```python
from build123d import *

# Parameters (mm, degrees)
SKETCH1_R           = 2.95
SKETCH1_R_2         = 1.9
BOSS_EXTRUDE1_DEPTH = 2
SKETCH2_R           = 0.5000000000000008
SKETCH2_R_2         = 0.75
BOSS_EXTRUDE2_DEPTH = 1.7


with BuildPart() as part:
    # Sketch1 → Boss-Extrude1 (new body)
    with BuildSketch(Plane(origin=(0, 0, 0), x_dir=(1, 0, 0), z_dir=(0, 1, 0))):
        with Locations(Location((0, 0, 0), (0, 0, 270))):
            Circle(SKETCH1_R)
        with Locations(Location((0, 0, 0), (0, 0, 270))):
            Circle(SKETCH1_R_2, mode=Mode.SUBTRACT)
    extrude(amount=BOSS_EXTRUDE1_DEPTH)

    # Sketch2 → Boss-Extrude2 (add)
    with BuildSketch(Plane(origin=(0, 2, 0), x_dir=(1, 0, 0), z_dir=(0, 1, 0))):
        with BuildLine():
            Line((-0.3719565217391307, 2.9264566195205663), (-11.689130434782609, 1.488028789586728))
            ThreePointArc((-11.689130434782609, 1.488028789586728), (-13, 1.8e-16), (-11.689130434782609, -1.488028789586728))
            Line((-11.689130434782609, -1.488028789586728), (-0.3719565217391307, -2.9264566195205663))
            ThreePointArc((-0.3719565217391307, -2.9264566195205663), (1.8e-16, -2.9500000000000024), (0.3719565217391307, -2.9264566195205663))
            Line((0.3719565217391307, -2.9264566195205663), (11.689130434782609, -1.488028789586728))
            ThreePointArc((11.689130434782609, -1.488028789586728), (13, 0), (11.689130434782609, 1.488028789586728))
            Line((11.689130434782609, 1.488028789586728), (0.3719565217391307, 2.9264566195205663))
            ThreePointArc((0.3719565217391307, 2.9264566195205663), (1.8e-16, 2.9500000000000024), (-0.3719565217391307, 2.9264566195205663))
        make_face()
        with Locations(Location((-11.5, 0, 0), (0, 0, 270))):
            Circle(SKETCH2_R, mode=Mode.SUBTRACT)
        with Locations(Location((-9.5, 0, 0), (0, 0, 270))):
            Circle(SKETCH2_R, mode=Mode.SUBTRACT)
        with Locations(Location((-7.5, 0, 0), (0, 0, 270))):
            Circle(SKETCH2_R, mode=Mode.SUBTRACT)
        with Locations(Location((7.5, 0, 0), (0, 0, 90))):
            Circle(SKETCH2_R, mode=Mode.SUBTRACT)
        with Locations(Location((9.5, 0, 0), (0, 0, 90))):
            Circle(SKETCH2_R, mode=Mode.SUBTRACT)
        with Locations(Location((11.5, 0, 0), (0, 0, 90))):
            Circle(SKETCH2_R, mode=Mode.SUBTRACT)
        with Locations(Location((0, 0, 0), (0, 0, 270))):
            Circle(SKETCH2_R_2, mode=Mode.SUBTRACT)
    extrude(amount=BOSS_EXTRUDE2_DEPTH)


solid = part.part
```
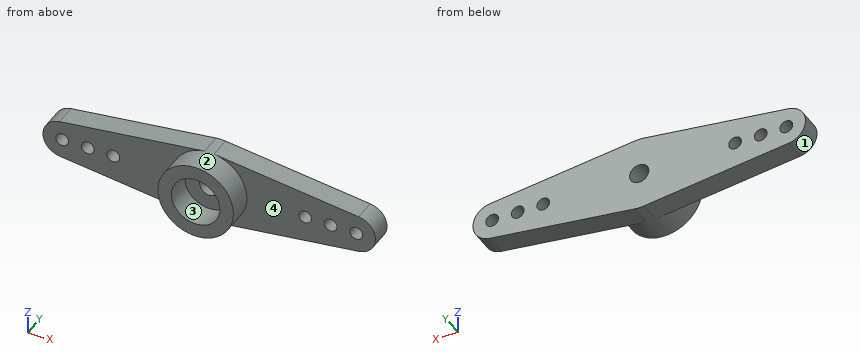
Part model, mm, in its own coordinate system. Face numbers are marked on the shaded views. Round coordinates to 2 decimals unless told otherwise and drop trailing zeros. Order: outer loops, then holes, each group sorted by start corner. A loop starts at its lowest first (then second) coordinate and runs counter-clockwise, first axis right, second up. Notation, with made-up numbers: M 39,71.25 L 66,71.25 A16 ccw 66,76.25 Z; hole C 27.5,15.25 d9. An arc over 180 degrees is marked long. Answer in a Markdown table with one row per item. Add a question column.
Q1. Mould opens along X. For the marked faces 1, 2, 3 and 4 say: +X half, -X half, draft (parallel to the pull), parting line (faces both ways), or undercut.
Q2. Pin check, flat tips, straight feed: pin 1 (1.2 mm diameter, centred on x = 0, z = 0, fed in from +Y); pin 2 (3 mm diameter, centred on x = 7, z = 1.5, fed in from -Y); pin 3 (2 mm diameter, centred on y = 1.5, z = 1, fed in from -X). Stop position of each tip, or through.
Q3. Cut at D-D on y = 1. Give the cut face in (x, z), and give its area (3 significant figures).
Q4. Cut at C-C on z = 2.5. Give the cut face in (x, y).
Q5. Cut at A-A on x = -7.5. Give the cut face in (y, z), and give its area (3 significant figures).
Q6. Wall check: L1, parallel to X at y = 1.65, z = 0; L2, parallel to Y at x = 7.75, z = 0.5; L3, parallel to Z at x = 11.5, y = 3. Give the ranges that are in metal, low to high. Write a range as from..to.
Q7. Cut at B-B on z = 0. Give the number of separate pieces and of enclosed holes in the cut face, and give its area (4 significant figures).
Established:
| question | item | result |
|---|---|---|
| 1 | face 1 | -X half |
| 1 | face 2 | parting line |
| 1 | face 3 | undercut |
| 1 | face 4 | draft |
| 2 | pin 1 | passes through |
| 2 | pin 2 | stops at y = 2 |
| 2 | pin 3 | stops at x = -12.99 |
| 3 | outline | C 0,0 d5.9; hole C 0,0 d3.8 |
| 3 | area | 16.0 mm2 |
| 4 | outline | M -3.73,2 L -1.57,2 L -1.57,0 L 1.57,0 L 1.57,2 L 3.73,2 L 3.73,3.7 L -3.73,3.7 Z |
| 5 | outline | M 2,-2.02 L 3.7,-2.02 L 3.7,-0.5 L 2,-0.5 Z; M 2,0.5 L 3.7,0.5 L 3.7,2.02 L 2,2.02 Z |
| 5 | area | 5.17 mm2 |
| 6 | L1 | x = -2.95..-1.9, 1.9..2.95 |
| 6 | L2 | y = 2..3.7 |
| 6 | L3 | z = -1.51..-0.5, 0.5..1.51 |
| 7 | separate pieces | 8 |
| 7 | enclosed holes | 0 |
| 7 | area | 35.65 mm2 |
